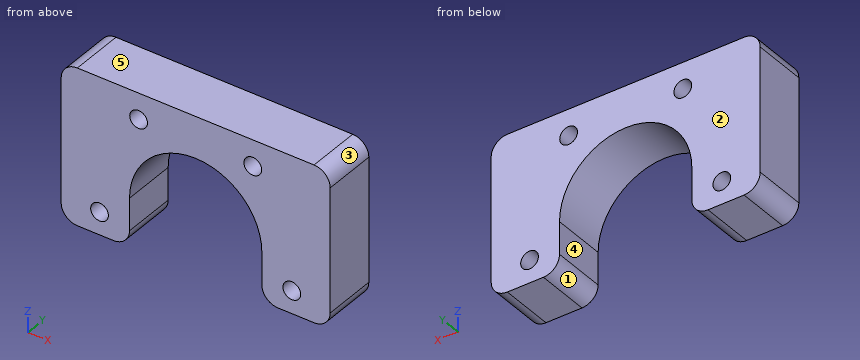
```python
from build123d import *

# Parameters (mm, degrees)
SKETCH_1_R      = 1.65
EXTRUDE_1_DEPTH = 10
FILLET_1_R      = 3


with BuildPart() as part:
    # 草图1 → 凸台-拉伸1 (new body)
    with BuildSketch(Plane(origin=(0, 0, 0), x_dir=(1, 0, 0), z_dir=(0, 1, 0))):
        with BuildLine():
            Line((-25, 30), (-25, 10))
            Line((-25, 10), (25, 10))
            Line((25, 10), (25, 30))
            Line((25, 30), (25, 39))
            Line((25, 39), (12.3, 39))
            Line((12.3, 39), (12.3, 30))
            ThreePointArc((12.3, 30), (0, 17.7), (-12.3, 30))
            Line((-12.3, 30), (-12.3, 39))
            Line((-12.3, 39), (-25, 39))
            Line((-25, 39), (-25, 30))
        make_face()
        with Locations(Location((-10.611164072, 14.845687181, 0), (0, 0, 270))):
            Circle(SKETCH_1_R, mode=Mode.SUBTRACT)
        with Locations(Location((-17.869627786, 34.788152334, 0), (0, 0, 270))):
            Circle(SKETCH_1_R, mode=Mode.SUBTRACT)
        with Locations(Location((10.611164072, 14.845687181, 0), (0, 0, 90))):
            Circle(SKETCH_1_R, mode=Mode.SUBTRACT)
        with Locations(Location((17.869627786, 34.788152334, 0), (0, 0, 90))):
            Circle(SKETCH_1_R, mode=Mode.SUBTRACT)
    extrude(amount=EXTRUDE_1_DEPTH)

    # 圆角1
    fillet_1_edges = [part.edges().sort_by_distance(p)[0] for p in [
        (25, 5, -10),
        (-25, 5, -10),
        (-25, 5, -39),
        (-12.3, 5, -39),
        (12.3, 5, -39),
        (25, 5, -39),
    ]]
    fillet(fillet_1_edges, radius=FILLET_1_R)


solid = part.part
```
The model under review builds one solid part; all positions refer to its coordinate system, in mm. Face numbers are marked on the shaded views. A direction names the side the tool comes from. Coordinates: 2 decimals unless noted, no trailing zeros. Write each loop counter-clockwise with the first axis right and the second up, starting at its lowest first coordinate (ties: lowest second). Pieces come first, ordered by that corner, then holes. Notation, with made-up numbers: (53, -13) - (70, -13) arc R26 cw to (70, 20) - close; hole circle Ø1 at (23.5, 54.25). An arc over 180 degrees is marked (long way). Answer in a Markdown table with one row per item. Add a question column.
Q1. For the marked faces 1 and 2, list the 3-axis set-ups (+Z, -Z, +X, -X, +Y, -Y) from which the entire face can be reached by the end or side of a thin tool; tool diameter is ignored.
Q2. Draft analysis for pull direction X (two halves, no side actions). For the marked faces 3, 4 and 5, state which applies: +X half, -X half, draft (parallel to the pull), parting line (faces both ways), or undercut.
Q3. Consider section A-A on z = -18.5. Give the boundary of the cut face in (x, y), then the cut area to 3 significant figures.
Q4. To check wall thickness, follow line 1 along X through (y, z) = (7.25, -14.25); line 2 along X through (y, z) = (4.5, -32.5); line 3 along X through (y, z) = (6.75, -35.75). State the ranges of each line that lie inside material, in increasing order. Write a range as from..to.
Q5. Consider section C-C on y = 8.5. Give the boundary of the cut face in (x, z).
Q6. Consider section D-D on z = -28.5. Give the boundary of the cut face in (x, y).
Q7. Consider section B-B on z = -14. Give the boundary of the cut face in (x, y), then the cut area to 3 significant figures.
Answers below:
| question | item | result |
|---|---|---|
| 1 | face 1 | -Z, +Y, -Y |
| 1 | face 2 | +Z, -Z, +X, -X, +Y |
| 2 | face 3 | +X half |
| 2 | face 4 | undercut |
| 2 | face 5 | draft |
| 3 | outline | (-25, 0) - (-4.36, 0) - (-4.36, 10) - (-25, 10) - close; (4.36, 0) - (25, 0) - (25, 10) - (4.36, 10) - close |
| 3 | area | 413 mm² |
| 4 | line 1 | -25..-12.15, -9.07..9.07, 12.15..25 |
| 4 | line 2 | -25..-12.3, 12.3..25 |
| 4 | line 3 | -25..-19.21, -16.53..-12.3, 12.3..16.53, 19.21..25 |
| 5 | outline | (-25, -36) arc R3 ccw to (-22, -39) - (-15.3, -39) arc R3 ccw to (-12.3, -36) - (-12.3, -30) arc R12.3 cw to (12.3, -30) - (12.3, -36) arc R3 ccw to (15.3, -39) - (22, -39) arc R3 ccw to (25, -36) - (25, -13) arc R3 ccw to (22, -10) - (-22, -10) arc R3 ccw to (-25, -13) - close; hole circle Ø3.3 at (-17.87, -34.79); hole circle Ø3.3 at (-10.61, -14.85); hole circle Ø3.3 at (10.61, -14.85); hole circle Ø3.3 at (17.87, -34.79) |
| 6 | outline | (-25, 0) - (-12.21, 0) - (-12.21, 10) - (-25, 10) - close; (12.21, 0) - (25, 0) - (25, 10) - (12.21, 10) - close |
| 7 | outline | (-25, 0) - (-12.03, 0) - (-12.03, 10) - (-25, 10) - close; (-9.19, 0) - (9.19, 0) - (9.19, 10) - (-9.19, 10) - close; (12.03, 0) - (25, 0) - (25, 10) - (12.03, 10) - close |
| 7 | area | 443 mm² |
